```python
from build123d import *

# Parameters (mm, degrees)
BOSS_EXTRU_1_DEPTH      = 100
ESQUISSE2_R             = 2.25
ENL_V_MAT_EXTRU_1_DEPTH = 11


with BuildPart() as part:
    # Esquisse1 → Boss.-Extru.1 (new body)
    with BuildSketch(Plane.XY):
        Polygon((-5.75, 0), (5.75, 0), (5.75, -10), (3.65, -10), (3.65, -3), (-3.65, -3), (-3.65, -10), (-5.75, -10), align=None)
    extrude(amount=-BOSS_EXTRU_1_DEPTH)

    # Esquisse2 → Enlèv. mat.-Extru.1 (cut, through all)
    with BuildSketch(Plane(origin=(0, 0, 0), x_dir=(1, 0, 0), z_dir=(0, 1, 0))):
        with Locations(Location((0, 86.5, 0), (0, 0, 270))):  # turned: the seam where the file's is
            Circle(ESQUISSE2_R)
        with Locations(Location((0, 13.5, 0), (0, 0, 270))):  # turned: the seam where the file's is
            Circle(ESQUISSE2_R)
        with BuildLine():
            Line((-3, 73.5), (-3, 41))
            ThreePointArc((-3, 41), (0, 38), (3, 41))
            Line((3, 41), (3, 73.5))
            ThreePointArc((3, 73.5), (0, 76.5), (-3, 73.5))
        make_face()
    extrude(amount=-ENL_V_MAT_EXTRU_1_DEPTH, mode=Mode.SUBTRACT)


solid = part.part
```
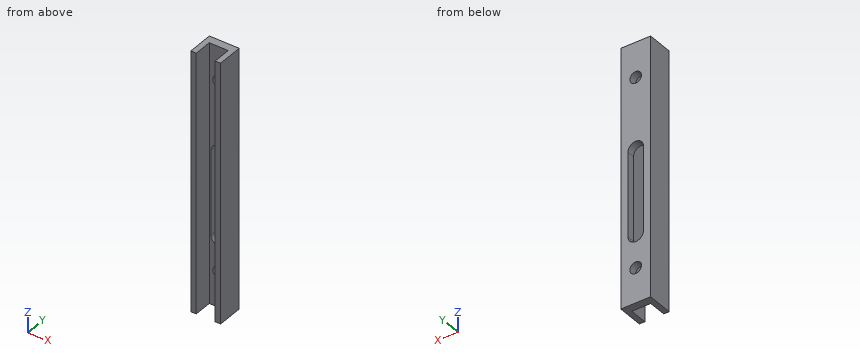
Here's how the part is built. I have some questions about the finished solid (model axes, mm). Coordinates: 2 decimals unless noted, no trailing zeros. Write each loop counter-clockwise with the first axis right and the second up, starting at its lowest first coordinate (ties: lowest second). Pieces come first, ordered by that corner, then holes. Notation, with made-up numbers: (45.5, -26.75) -> (69.5, -26.75) arc R16 ccw to (69.5, -22.75) -> close; hole circle Ø1 at (58, -31). An arc over 180 degrees is marked (long way). Use a Markdown table: item, result. Add a question column.
(1) If we section it at C-C, the plane x = 0: Write out the boundary of the cut face in (y, z), and give its area (4 significant figures).
(2) If we section it at A-A, the plane z = -64.5: Write out the boundary of the cut face in (x, y), and give its area (3 significant figures).
(3) If we section it at B-B, the plane y = -4.5: Write out the boundary of the cut face in (x, z).
(4) I'm going to push flat-ended pins straight in: P1, Ø5, axis at x = 1, z = -51, coming from the -Y side; P2, Ø4, axis at x = 0, z = -13.5, coming from the +Y side. Where does each tip first touch, or does it pass through?
(5) If we section it at D-D, the plane z = -22: Write out the boundary of the cut face in (x, y).
(6) Please list where these lines run through material, in increasing order: line 1 (X direction, y = -8.5, z = -42); line 2 (X direction, y = -1.7, z = -13.5); line 3 (Y direction, x = 1, z = -79.5).
Outcome:
| question | item | result |
|---|---|---|
| 1 | outline | (-3, -100) -> (0, -100) -> (0, -88.75) -> (-3, -88.75) -> close; (-3, -84.25) -> (0, -84.25) -> (0, -76.5) -> (-3, -76.5) -> close; (-3, -38) -> (0, -38) -> (0, -15.75) -> (-3, -15.75) -> close; (-3, -11.25) -> (0, -11.25) -> (0, 0) -> (-3, 0) -> close |
| 1 | area | 157.5 mm^2 |
| 2 | outline | (-5.75, -10) -> (-3.65, -10) -> (-3.65, -3) -> (-3, -3) -> (-3, 0) -> (-5.75, 0) -> close; (3, -3) -> (3.65, -3) -> (3.65, -10) -> (5.75, -10) -> (5.75, 0) -> (3, 0) -> close |
| 2 | area | 45.9 mm^2 |
| 3 | outline | (-5.75, -100) -> (-3.65, -100) -> (-3.65, 0) -> (-5.75, 0) -> close; (3.65, -100) -> (5.75, -100) -> (5.75, 0) -> (3.65, 0) -> close |
| 4 | P1 | stops at y = -3 |
| 4 | P2 | passes through |
| 5 | outline | (-5.75, -10) -> (-3.65, -10) -> (-3.65, -3) -> (3.65, -3) -> (3.65, -10) -> (5.75, -10) -> (5.75, 0) -> (-5.75, 0) -> close |
| 6 | line 1 | x = -5.75 to -3.65, 3.65 to 5.75 |
| 6 | line 2 | x = -5.75 to -2.25, 2.25 to 5.75 |
| 6 | line 3 | y = -3 to 0 |
